Build history of the part. All positions in model axes, mm. Round coordinates to 2 decimals unless told otherwise and drop trailing zeros. Write each loop counter-clockwise with the first axis right and the second up, starting at its lowest first coordinate (ties: lowest second). Pieces come first, ordered by that corner, then holes.
Item 1: Drop flat-ended pins along their axis: pin 1 Ø2.5 at (x, y) = (126.5, 2) entering from +Z; pin 2 Ø2 at (y, z) = (3.5, 2.5) entering from +X; pin 3 Ø1.3 at (y, z) = (1.5, -9.5) entering from -X; pin 4 Ø2 at (x, z) = (4.35, -41.65) entering from -Y. Give the stop position or say it passes through.
Item 2: Band-saw the part on D-D, the plane x = 28.5. Write the cut outline in (y, z).
Item 3: Wall check: probe 1 along X at (y, z) = (3.25, -25.5); probe 2 along X at (y, z) = (1.2, -4); probe 3 along Z at (x, y) = (165.65, 2.8). Give the ranges that are in metal, low to high.
Item 4: Band-saw the part on C-C, the plane y = 3.1. Count the separate pieces of the cut face and the enclosed holes in it, then the cut area to 3 significant figures.
Item 5: Band-saw the part on B-B, the plane z = -25. Write the cut outline in (x, y), then the cut area to 3 significant figures.
Item 6: Band-saw the part on A-A, the plane x = 155. Write the cut outline in (y, z).
```python
from build123d import *

# Parameters (mm, degrees)
SKETCH_1_W          = 170
SKETCH_1_H          = 52
EXTRUDE_1_DEPTH     = 5
SKETCH_2_R          = 11.5
SKETCH_2_R_2        = 1.75
CUT_EXTRUDE_1_DEPTH = 5
SKETCH_3_W          = 20
SKETCH_3_H          = 5
EXTRUDE_2_DEPTH     = 5
SKETCH_4_R          = 1
CUT_EXTRUDE_2_DEPTH = 5
CUT_EXTRUDE_3_DEPTH = 10
FILLET_1_R          = 0.5
SKETCH_7_W          = 3
SKETCH_7_H          = 32
EXTRUDE_3_DEPTH     = 5
SKETCH_8_R          = 1
CUT_EXTRUDE_5_DEPTH = 5
SKETCH_9_W          = 80
SKETCH_9_H          = 40
CUT_EXTRUDE_6_DEPTH = 10
FILLET_2_R          = 1.5
FILLET_3_R          = 1


with BuildPart() as part:
    # 스케치1 → 보스-돌출1 (new body)
    with BuildSketch(Plane(origin=(0, 0, 0), x_dir=(1, 0, 0), z_dir=(0, 1, 0))):
        with Locations((85, 26)):
            Rectangle(SKETCH_1_W, SKETCH_1_H)
    extrude(amount=EXTRUDE_1_DEPTH)

    # 스케치2 → 컷-돌출1 (cut)
    with BuildSketch(Plane(origin=(0, 5, 0), x_dir=(1, 0, 0), z_dir=(0, 1, 0))):
        with Locations(Location((150, 26, 0), (0, 0, 270))):
            Circle(SKETCH_2_R)
        with Locations(Location((165.65, 41.65, 0), (0, 0, 270))):
            Circle(SKETCH_2_R_2)
        with Locations(Location((134.35, 41.65, 0), (0, 0, 270))):
            Circle(SKETCH_2_R_2)
        with Locations(Location((165.65, 10.35, 0), (0, 0, 270))):
            Circle(SKETCH_2_R_2)
        with Locations(Location((134.35, 10.35, 0), (0, 0, 270))):
            Circle(SKETCH_2_R_2)
        with Locations(Location((35.65, 10.35, 0), (0, 0, 90))):
            Circle(SKETCH_2_R_2)
        with Locations(Location((4.35, 10.35, 0), (0, 0, 90))):
            Circle(SKETCH_2_R_2)
        with Locations(Location((35.65, 41.65, 0), (0, 0, 90))):
            Circle(SKETCH_2_R_2)
        with Locations(Location((4.35, 41.65, 0), (0, 0, 90))):
            Circle(SKETCH_2_R_2)
        with Locations(Location((20, 26, 0), (0, 0, 90))):
            Circle(SKETCH_2_R)
    extrude(amount=-CUT_EXTRUDE_1_DEPTH, mode=Mode.SUBTRACT)

    # 스케치3 → 보스-돌출2 (add)
    with BuildSketch(Plane(origin=(0, 5, 0), x_dir=(1, 0, 0), z_dir=(0, 1, 0))):
        with Locations((140, -2.5)):
            Rectangle(SKETCH_3_W, SKETCH_3_H)
        with Locations((30, -2.5)):
            Rectangle(SKETCH_3_W, SKETCH_3_H)
    extrude(amount=-EXTRUDE_2_DEPTH)

    # 스케치4 → 컷-돌출2 (cut)
    with BuildSketch(Plane(origin=(0, 5, 0), x_dir=(1, 0, 0), z_dir=(0, 1, 0))):
        with Locations((129, 0)):
            Circle(SKETCH_4_R)
        with Locations((151, 0)):
            Circle(SKETCH_4_R)
        with Locations((19, 0)):
            Circle(SKETCH_4_R)
        with Locations((41, 0)):
            Circle(SKETCH_4_R)
    extrude(amount=-CUT_EXTRUDE_2_DEPTH, mode=Mode.SUBTRACT)

    # 스케치5 → 컷-돌출3 (cut)
    with BuildSketch(Plane(origin=(0, 5, 0), x_dir=(1, 0, 0), z_dir=(0, 1, 0))):
        with BuildLine():
            Line((156.55, 0), (156.55, 6))
            Line((156.55, 6), (157.75, 6))
            ThreePointArc((157.75, 6), (159.15, 7.4), (157.75, 8.8))
            Line((157.75, 8.8), (156.55, 8.8))
            Line((156.55, 8.8), (156.55, 10))
            ThreePointArc((156.55, 10), (155, 11.55), (153.45, 10))
            Line((153.45, 10), (153.45, 8.8))
            Line((153.45, 8.8), (152.25, 8.8))
            ThreePointArc((152.25, 8.8), (150.85, 7.4), (152.25, 6))
            Line((152.25, 6), (153.45, 6))
            Line((153.45, 6), (153.45, 0))
            Line((153.45, 0), (156.55, 0))
        make_face()
        with BuildLine():
            Line((12.25, 6), (13.45, 6))
            Line((13.45, 6), (13.45, 0))
            Line((13.45, 0), (16.55, 0))
            Line((16.55, 0), (16.55, 6))
            Line((16.55, 6), (17.75, 6))
            ThreePointArc((17.75, 6), (19.15, 7.4), (17.75, 8.8))
            Line((17.75, 8.8), (16.55, 8.8))
            Line((16.55, 8.8), (16.55, 10))
            ThreePointArc((16.55, 10), (15, 11.55), (13.45, 10))
            Line((13.45, 10), (13.45, 8.8))
            Line((13.45, 8.8), (12.25, 8.8))
            ThreePointArc((12.25, 8.8), (10.85, 7.4), (12.25, 6))
        make_face()
    extrude(amount=-CUT_EXTRUDE_3_DEPTH, mode=Mode.SUBTRACT)

    # 필렛1
    fillet_1_edges = [part.edges().sort_by_distance(p)[0] for p in [
        (20, 2.5, 5),
        (130, 2.5, 5),
        (150, 2.5, 5),
        (40, 2.5, 5),
    ]]
    fillet(fillet_1_edges, radius=FILLET_1_R)

    # 스케치7 → 보스-돌출3 (add)
    with BuildSketch(Plane(origin=(0, 5, 0), x_dir=(1, 0, 0), z_dir=(0, 1, 0))):
        with Locations((171.5, 36)):
            Rectangle(SKETCH_7_W, SKETCH_7_H)
        with Locations((-1.5, 36)):
            Rectangle(SKETCH_7_W, SKETCH_7_H)
    extrude(amount=-EXTRUDE_3_DEPTH)

    # 스케치8 → 컷-돌출5 (cut)
    with BuildSketch(Plane(origin=(0, 5, 0), x_dir=(1, 0, 0), z_dir=(0, 1, 0))):
        with Locations((170, 19)):
            Circle(SKETCH_8_R)
        with Locations((0, 19)):
            Circle(SKETCH_8_R)
    extrude(amount=-CUT_EXTRUDE_5_DEPTH, mode=Mode.SUBTRACT)

    # 스케치9 → 컷-돌출6 (cut)
    with BuildSketch(Plane(origin=(0, 5, 0), x_dir=(1, 0, 0), z_dir=(0, 1, 0))):
        with Locations((85, 20)):
            Rectangle(SKETCH_9_W, SKETCH_9_H)
    extrude(amount=-CUT_EXTRUDE_6_DEPTH, mode=Mode.SUBTRACT)

    # 필렛2
    fillet_2_edges = [part.edges().sort_by_distance(p)[0] for p in [
        (125, 2.5, -40),
        (45, 2.5, -40),
    ]]
    fillet(fillet_2_edges, radius=FILLET_2_R)

    # 필렛3
    fillet_3_edges = [part.edges().sort_by_distance(p)[0] for p in [
        (173, 2.5, -20),
        (-3, 2.5, -20),
    ]]
    fillet(fillet_3_edges, radius=FILLET_3_R)


solid = part.part
```
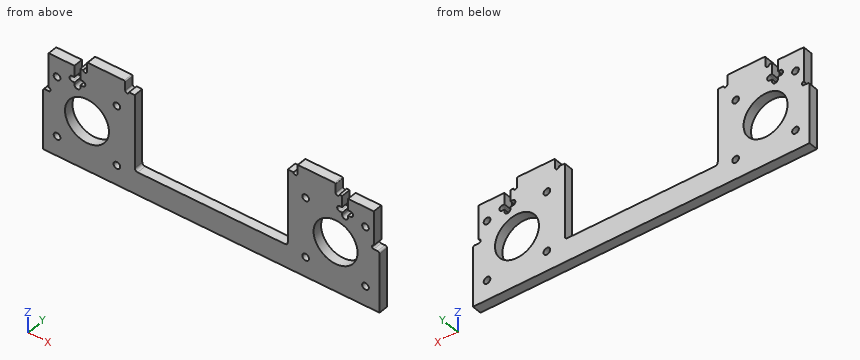
Results:
1. pin 1: stops at z = 0
1. pin 2: stops at x = 150
1. pin 3: stops at x = 0
1. pin 4: passes through
2. outline: (0, -52) - (5, -52) - (5, -33.75) - (0, -33.75) - close; (0, -18.25) - (5, -18.25) - (5, 5) - (0, 5) - close
3. probe 1: x = -3 to 8.51, 31.49 to 45, 125 to 138.51, 161.49 to 173
3. probe 2: x = 0 to 13.45, 16.55 to 45, 125 to 153.45, 156.55 to 170
3. probe 3: z = -52 to -43.4, -39.9 to -12.1, -8.6 to 0
4. separate pieces: 1
4. enclosed holes: 10
4. area: 5,020 mm2
5. outline: (-3, 0) - (8.54, 0) - (8.54, 5) - (-3, 5) - close; (31.46, 0) - (45, 0) - (45, 5) - (31.46, 5) - close; (125, 0) - (138.54, 0) - (138.54, 5) - (125, 5) - close; (161.46, 0) - (173, 0) - (173, 5) - (161.46, 5) - close
5. area: 251 mm2
6. outline: (0, -52) - (5, -52) - (5, -36.36) - (0, -36.36) - close; (0, -15.64) - (5, -15.64) - (5, -11.55) - (0, -11.55) - close
